Autodesk Inventor part; units mm, degrees
ref_plane "YZ Plane" through (0, 0, 0) normal (1, 0, 0) x (0, 1, 0)
ref_plane "XZ Plane" through (0, 0, 0) normal (0, 1, 0) x (-1, 0, 0)
ref_plane "XY Plane" through (0, 0, 0) normal (0, 0, 1) x (1, 0, 0)
sketch "Sketch1" plane through (0, 0, 0) normal (0, 0, 1) x (1, 0, 0)
  line L0 (-10, -10) -> (10, -10)
  line L1 (10, -10) -> (10, 10)
  line L2 (10, 10) -> (-10, 10)
  line L3 (-10, 10) -> (-10, -10)
  line L4 (-10, -10) -> (10, 10) construction
  line L5 (10, -10) -> (-10, 10) construction
  point P0 (0, 0)
  dimension "d0" = 20
  dimension "d1" = 20
extrude "Extrusion1" add sketch "Sketch1" along normal blind 30
sketch "Sketch2" plane through (0, 0, 0) normal (0, 0, -1) x (-1, 0, 0)
  point P0 (0, 0)
  point P1 (-8, 8)
  point P2 (8, 8)
  point P3 (8, -8)
  point P4 (-8, -8)
  dimension "d4" = 8
  dimension "d5" = 8
  dimension "d6" = 8
  dimension "d7" = 8
  dimension "d8" = 8
  dimension "d9" = 8
  dimension "d10" = 8
  dimension "d11" = 8
hole "Hole1" at (8, 8, 0) at (-8, 8, 0) at (-8, -8, 0) at (8, -8, 0) direction (0, 0, 1) diameter 2 depth 3.5 tip angle 118
sketch "Sketch3" plane through (0, 0, 0) normal (0, 0, -1) x (-1, 0, 0)
  circle A0 centre (0, 0) radius 7.5
  dimension "d19" = 15
extrude "Extrusion2" add sketch "Sketch3" along normal blind 1.5
sketch "Sketch4" plane through (0, 0, -1.5) normal (0, 0, -1) x (-1, 0, 0)
  circle A0 centre (0, 0) radius 7.5
  circle A1 centre (0, 0) radius 2
  dimension "d22" = 4
extrude "Extrusion3" add sketch "Sketch4" along normal blind 13.5 contours A1
properties part number "NEMA8"
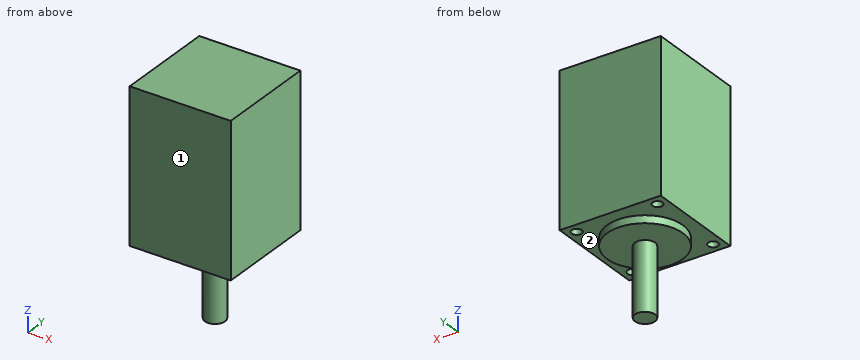
Input: part model. Units: mm. Frame: model coordinates. Face numbers are marked on the shaded views. A direction names the side the tool comes from. Round coordinates to 2 decimals unless told otherwise and drop trailing zeros. Order: outer loops, then holes, each group sorted by start corner. A loop starts at its lowest first (then second) coordinate and runs counter-clockwise, first axis right, second up.
1. Cut plane A-A, the plane x = -4.5. Output: boundary loops of the cut face in (y, z).
The answers:
outline: (-10, 0) - (-6, 0) - (-6, -1.5) - (6, -1.5) - (6, 0) - (10, 0) - (10, 30) - (-10, 30) - close
2. Material intervals for line 1 (Y direction, x = 8, z = 2.8); line 2 (Z direction, x = 9.25, y = -4.25), sorted ascending.
The answers:
line 1: y = -10 to -9, -7 to 7, 9 to 10
line 2: z = 0 to 30
3. Set-up query: the marked faces 1 and 2. Return all of +Z, -Z, +X, -X, +Y, -Y with unobstructed straight access to the full face (end or side cutting, diameter ignored); none if empty.
The answers:
face 1: +Z, -Z, +X, -X, -Y
face 2: -Z
4. Pin query (flat end, axial travel): P1, Ø12, axis at x = -3, y = 0, coming from the -Z side; P2, Ø10, axis at y = 4, z = -5.5, coming from the +X side; P3, Ø1.2, axis at x = 8, y = -8, coming from the -Z side; P4, Ø3, axis at x = 8, y = 8, coming from the -Z side. Return the tip coordinate at first contact, or that it passes through.
The answers:
P1: stops at z = -15
P2: stops at x = 7.43
P3: stops at z = 3.74
P4: stops at z = 0
5. Cut plane C-C, the plane z = 1. Output: boundary loops of the cut face in (x, y), then the cut area to 3 significant figures.
The answers:
outline: (-10, -10) - (10, -10) - (10, 10) - (-10, 10) - close; hole circle Ø2 at (-8, -8); hole circle Ø2 at (-8, 8); hole circle Ø2 at (8, -8); hole circle Ø2 at (8, 8)
area: 387 mm2
6. Cut plane B-B, the plane y = 0. Output: boundary loops of the cut face in (x, z), then the cut area to 4 significant figures.
The answers:
outline: (-10, 0) - (-7.5, 0) - (-7.5, -1.5) - (-2, -1.5) - (-2, -15) - (2, -15) - (2, -1.5) - (7.5, -1.5) - (7.5, 0) - (10, 0) - (10, 30) - (-10, 30) - close
area: 676.5 mm2
